```python
from build123d import *

# Parameters (mm, degrees)
BOSS_EXTRUDE1_DEPTH = 12.7


with BuildPart() as part:
    # Sketch1 → Boss-Extrude1 (new body)
    with BuildSketch(Plane.XY):
        with BuildLine():
            Line((-38.1, -19.05), (38.1, -19.05))
            Line((38.1, -19.05), (38.1, 0))
            Line((38.1, 0), (14.605, 0))
            ThreePointArc((14.605, 0), (0, -14.605), (-14.605, 0))
            Line((-14.605, 0), (-38.1, 0))
            Line((-38.1, 0), (-38.1, -19.05))
        make_face()
    extrude(amount=BOSS_EXTRUDE1_DEPTH)


solid = part.part
```
Source: CAD feature listing. Evaluate the final solid. Frame: model axes, mm. Coordinates: 2 decimals unless noted, no trailing zeros. Loops run counter-clockwise (first coordinate to the right, second up) from the corner with the lowest first, then second, coordinate; pieces in that order, holes last. Notation, with made-up numbers: M -39,39 L -15,39 A16 cw -15,50 Z; hole C 15.5,48 d7. An arc over 180 degrees is marked long. Put each result on its own line as item: value. Start each with the question number.
1) Pull-direction query (X, two-part tool) for faces 1 (the face through (-1, -16, 0)), 2 (the face through (-38.1, -9, 6)), 3 (the face through (0.3, -14.6, 6.3)), 4 (the face through (38.1, -10, 6)); classes: pulls with the +X half, pulls with the -X half, needs draft (parallel to the pull), parting line crosses it, or undercut.
2) Cut plane C-C on y = -9.25. Return the cut outline in (x, z), then the cut area to 3 significant figures.
3) Cut plane B-B on z = 1. Return the cut outline in (x, y) (3 decimals), then the cut area to 3 significant figures.
4) Ray query, L1, parallel to X at y = -11, z = 7; L2, parallel to X at y = -7.25, z = 11.75; L3, parallel to Y at x = -4, z = 3. Return the intervals inside material, ascending. Write a range as from..to.
5) Contact query for a flat-ended pin moving along its axis: pin 1 Ø1 at (x, z) = (2, 10) entering from +Y. Output: stop coordinate, or through.
6) Cut plane D-D on x = 0. Return the cut outline in (y, z) (3 decimals).
7) Cut plane A-A on y = -12.25. Return the cut outline in (x, z).
The answers:
1. face 1: needs draft
1. face 2: pulls with the -X half
1. face 3: undercut
1. face 4: pulls with the +X half
2. outline: M -38.1,0 L -11.3,0 L -11.3,12.7 L -38.1,12.7 Z; M 11.3,0 L 38.1,0 L 38.1,12.7 L 11.3,12.7 Z
2. area: 681 mm²
3. outline: M -38.1,-19.05 L 38.1,-19.05 L 38.1,0 L 14.605,0 A14.605 cw -14.605,0 L -38.1,0 Z
3. area: 1,120 mm²
4. L1: x = -38.1..-9.61, 9.61..38.1
4. L2: x = -38.1..-12.68, 12.68..38.1
4. L3: y = -19.05..-14.05
5. pin 1: stops at y = -14.39
6. outline: M -19.05,0 L -14.605,0 L -14.605,12.7 L -19.05,12.7 Z
7. outline: M -38.1,0 L -7.95,0 L -7.95,12.7 L -38.1,12.7 Z; M 7.95,0 L 38.1,0 L 38.1,12.7 L 7.95,12.7 Z
